from build123d import *

# Parameters (mm, degrees)
SKETCH_1_R               = 10
EXTRUDE_1_DEPTH          = 20
CUT_EXTRUDE_1_DEPTH      = 55.598534779
CUT_EXTRUDE_1_DEPTH_BACK = 55.598534779
SKETCH_2_R               = 3.3


with BuildPart() as part:
    # 草图1 → 凸台-拉伸1 (new body)
    with BuildSketch(Plane.XY):
        Polygon((-15, 51), (15, 51), (15, 10), (30, 10), (30, 0), (-30, 0), (-30, 10), (-15, 10), align=None)
        with Locations((0, 31)):
            Circle(SKETCH_1_R, mode=Mode.SUBTRACT)
    extrude(amount=EXTRUDE_1_DEPTH)

    # 草图2 → 切除-拉伸1 (cut, two sides: drawn at the far end of the back side and taken through both)
    with BuildSketch(Plane(origin=(0, 10, 0), x_dir=(1, 0, 0), z_dir=(0, 1, 0)).offset(-CUT_EXTRUDE_1_DEPTH_BACK)):
        with Locations(Location((-22.5, -10, 0), (0, 0, 180))):
            Circle(SKETCH_2_R)
        with Locations(Location((22.5, -10, 0), (0, 0, 90))):
            Circle(SKETCH_2_R)
    extrude(amount=CUT_EXTRUDE_1_DEPTH + CUT_EXTRUDE_1_DEPTH_BACK, mode=Mode.SUBTRACT)


solid = part.part
Design review of the part built by this model. Coordinates are the model's own, in mm. A direction names the side the tool comes from. Round coordinates to 2 decimals unless told otherwise and drop trailing zeros. Write each loop counter-clockwise with the first axis right and the second up, starting at its lowest first coordinate (ties: lowest second). Pieces come first, ordered by that corner, then holes. Notation, with made-up numbers: (71, 14.25) - (117, 14.25) arc R31 ccw to (117, 41.25) - close; hole circle Ø9 at (9.25, -32). An arc over 180 degrees is marked (long way). Use a Markdown table: item, result. Add a question column.
1. We need section B-B (x = 22.5). State the section outline as (y, z) points.
2. Wall thickness on probe 1 along X at (y, z) = (7.75, 10); probe 2 along Z at (x, y) = (-22.5, 5.25); probe 3 along Y at (x, z) = (-23, 3): over which ranges is each line inside the solid? List them lowest first.
3. We need section A-A (y = 31). State the section outline as (x, z) points, then the cut area to 3 significant figures.
4. For faces 1 (the face through (0, 0, 10)), 2 (the face through (-26, 10, 10)), 3 (the face through (19, 10, 10)), list the 3-axis set-ups (+Z, -Z, +X, -X, +Y, -Y) from which the entire face can be reached by the end or side of a thin tool; tool diameter is ignored.
5. Mouldability with a two-part tool opening along Z and no side actions: class faces 4 (the face through (0, 20, 0)), 5 (the face through (24.508, 4.93, 12.619)), 6 (the face through (-15, 30, 10)), 7 (the face through (-25.55, 4.93, 8.74)) as +Z half, -Z half, draft (parallel to the pull), parting line (faces both ways), or undercut.
6. We need section D-D (z = 10.75). State the section outline as (x, y) points.
7. Clearance check with flat-ended pins moving along their axes: pin 1 (6 mm diameter, centred on x = 22.5, z = 10, fed in from -Y); pin 2 (8 mm diameter, centred on y = 25, z = 12.5, fed in from +X); pin 3 (1 mm diameter, centred on y = 26, z = 15.5, fed in from -X). State where each tip first meets the part, or that it passes through.
8. We need section C-C (z = 17). State the section outline as (x, y) points.
Output:
| question | item | result |
|---|---|---|
| 1 | outline | (0, 0) - (10, 0) - (10, 6.7) - (0, 6.7) - close; (0, 13.3) - (10, 13.3) - (10, 20) - (0, 20) - close |
| 2 | probe 1 | x = -30 to -25.8, -19.2 to 19.2, 25.8 to 30 |
| 2 | probe 2 | z = 0 to 6.7, 13.3 to 20 |
| 2 | probe 3 | y = 0 to 10 |
| 3 | outline | (-15, 0) - (-10, 0) - (-10, 20) - (-15, 20) - close; (10, 0) - (15, 0) - (15, 20) - (10, 20) - close |
| 3 | area | 200 mm2 |
| 4 | face 1 | +Z, -Z, +X, -X, -Y |
| 4 | face 2 | +Z, -Z, -X, +Y |
| 4 | face 3 | +Z, -Z, +X, +Y |
| 5 | face 4 | -Z half |
| 5 | face 5 | undercut |
| 5 | face 6 | draft |
| 5 | face 7 | undercut |
| 6 | outline | (-30, 0) - (-25.71, 0) - (-25.71, 10) - (-30, 10) - close; (-19.29, 0) - (19.29, 0) - (19.29, 10) - (15, 10) - (15, 51) - (-15, 51) - (-15, 10) - (-19.29, 10) - close; (25.71, 0) - (30, 0) - (30, 10) - (25.71, 10) - close; hole circle Ø20 at (0, 31) |
| 7 | pin 1 | passes through |
| 7 | pin 2 | stops at x = 15 |
| 7 | pin 3 | stops at x = -15 |
| 8 | outline | (-30, 0) - (30, 0) - (30, 10) - (15, 10) - (15, 51) - (-15, 51) - (-15, 10) - (-30, 10) - close; hole circle Ø20 at (0, 31) |
